from build123d import *

# Parameters (mm, degrees)
MODEL_W                      = 31.7
MODEL_H                      = 20.375
SALIENTE_EXTRUIR1_DEPTH      = 4
SALIENTE_EXTRUIR2_DEPTH      = 4
SALIENTE_EXTRUIR2_DEPTH_BACK = 4
CROQUIS3_W                   = 37.7
CROQUIS3_H                   = 26.375
CROQUIS3_W_2                 = 31.7
CROQUIS3_H_2                 = 20.375
REDONDEO1_R                  = 5
REDONDEO3_R                  = 5
CROQUIS8_W                   = 31.7
CROQUIS8_H                   = 3.000145556
CORTAR_EXTRUIR2_DEPTH        = 4
CORTAR_EXTRUIR3_DEPTH        = 4
CHAFL_N3_SIZE                = 1.5
CHAFL_N4_SIZE                = 1


with BuildPart() as part:
    # Model → Saliente-Extruir1 (new body)
    with BuildSketch(Plane.XY):
        with Locations((126.95, -64.0625)):
            Rectangle(MODEL_W, MODEL_H)
        Polygon((126.809569, -61.253776), (127.077015, -61.28391), (127.339405, -61.343798), (127.59344, -61.432689), (127.835925, -61.549464), (128.063811, -61.692654), (128.274232, -61.860459), (128.464541, -62.050768), (128.632346, -62.261189), (128.775536, -62.489075), (128.892311, -62.73156), (128.981202, -62.985595), (129.04109, -63.247985), (129.071224, -63.515431), (129.071224, -63.784569), (129.04109, -64.052015), (128.981202, -64.314405), (128.892311, -64.56844), (128.775536, -64.810925), (128.632346, -65.038811), (128.464541, -65.249232), (128.274232, -65.439541), (128.063811, -65.607346), (127.835925, -65.750536), (127.59344, -65.867311), (127.339405, -65.956202), (127.077015, -66.01609), (126.809569, -66.046224), (126.540431, -66.046224), (126.272985, -66.01609), (126.010595, -65.956202), (125.75656, -65.867311), (125.514075, -65.750536), (125.286189, -65.607346), (125.075768, -65.439541), (124.885459, -65.249232), (124.717654, -65.038811), (124.574464, -64.810925), (124.457689, -64.56844), (124.368798, -64.314405), (124.30891, -64.052015), (124.278776, -63.784569), (124.278776, -63.515431), (124.279861, -63.505804), (124.30891, -63.247985), (124.368798, -62.985595), (124.457689, -62.73156), (124.574464, -62.489075), (124.717654, -62.261189), (124.885459, -62.050768), (125.075768, -61.860459), (125.286189, -61.692654), (125.514075, -61.549464), (125.75656, -61.432689), (126.010595, -61.343798), (126.272985, -61.28391), (126.540431, -61.253776), align=None, mode=Mode.SUBTRACT)
    extrude(amount=SALIENTE_EXTRUIR1_DEPTH)

    # Croquis3 → Saliente-Extruir2 (add, two sides: drawn at the far end of the back side and taken through both)
    with BuildSketch(Plane.XY.offset(4).offset(-SALIENTE_EXTRUIR2_DEPTH_BACK)):
        with Locations((126.95, -64.0625)):
            Rectangle(CROQUIS3_W, CROQUIS3_H)
        with Locations((126.95, -64.0625)):
            Rectangle(CROQUIS3_W_2, CROQUIS3_H_2, mode=Mode.SUBTRACT)
    extrude(amount=SALIENTE_EXTRUIR2_DEPTH + SALIENTE_EXTRUIR2_DEPTH_BACK)

    # Redondeo1
    redondeo1_edges = [part.edges().sort_by_distance(p)[0] for p in [
        (108.1, -77.25, 4),
        (145.8, -77.25, 4),
    ]]
    fillet(redondeo1_edges, radius=REDONDEO1_R)

    # Redondeo3
    redondeo3_edges = [part.edges().sort_by_distance(p)[0] for p in [
        (145.8, -50.875, 4),
        (108.1, -50.875, 4),
    ]]
    fillet(redondeo3_edges, radius=REDONDEO3_R)

    # Croquis8 → Cortar-Extruir2 (cut)
    with BuildSketch(Plane.XZ.offset(53.875)):
        with Locations((126.95, 6.499927222)):
            Rectangle(CROQUIS8_W, CROQUIS8_H)
    extrude(amount=-CORTAR_EXTRUIR2_DEPTH, mode=Mode.SUBTRACT)

    # Croquis9 → Cortar-Extruir3 (cut)
    with BuildSketch(Plane.XY.offset(4)):
        with BuildLine():
            Line((115.1, -56.375), (118.625993534, -56.375))
            Line((118.625993534, -56.375), (122.824085816, -56.375))
            ThreePointArc((122.824085816, -56.375), (123.884745987, -56.814339828), (124.324085816, -57.875))
            Line((124.324085816, -57.875), (124.324085816, -58.116279303))
            ThreePointArc((124.324085816, -58.116279303), (123.884745987, -59.176939475), (122.824085816, -59.616279303))
            Line((122.824085816, -59.616279303), (118.862646904, -59.616279303))
            ThreePointArc((118.862646904, -59.616279303), (117.801986732, -60.055619131), (117.362646904, -61.116279303))
            Line((117.362646904, -61.116279303), (117.362646904, -70.15))
            ThreePointArc((117.362646904, -70.15), (116.923307076, -71.210660172), (115.862646904, -71.65))
            Line((115.862646904, -71.65), (115.1, -71.65))
            ThreePointArc((115.1, -71.65), (114.039339828, -71.210660172), (113.6, -70.15))
            Line((113.6, -70.15), (113.6, -57.875))
            ThreePointArc((113.6, -57.875), (114.039339828, -56.814339828), (115.1, -56.375))
        make_face()
        with BuildLine():
            Line((138.8, -71.65), (138.037353096, -71.65))
            ThreePointArc((138.037353096, -71.65), (136.976692924, -71.210660172), (136.537353096, -70.15))
            Line((136.537353096, -70.15), (136.537353096, -63.375))
            ThreePointArc((136.537353096, -63.375), (136.976692924, -62.314339828), (138.037353096, -61.875))
            Line((138.037353096, -61.875), (138.8, -61.875))
            ThreePointArc((138.8, -61.875), (139.860660172, -62.314339828), (140.3, -63.375))
            Line((140.3, -63.375), (140.3, -70.15))
            ThreePointArc((140.3, -70.15), (139.860660172, -71.210660172), (138.8, -71.65))
        make_face()
        with BuildLine():
            Line((130.618924081, -56.194062707), (135.761102268, -56.194062707))
            ThreePointArc((135.761102268, -56.194062707), (136.82176244, -56.633402535), (137.261102268, -57.694062707))
            Line((137.261102268, -57.694062707), (137.261102268, -57.771184154))
            ThreePointArc((137.261102268, -57.771184154), (136.82176244, -58.831844326), (135.761102268, -59.271184154))
            Line((135.761102268, -59.271184154), (130.618924081, -59.271184154))
            ThreePointArc((130.618924081, -59.271184154), (129.55826391, -58.831844326), (129.118924081, -57.771184154))
            Line((129.118924081, -57.771184154), (129.118924081, -57.694062707))
            ThreePointArc((129.118924081, -57.694062707), (129.55826391, -56.633402535), (130.618924081, -56.194062707))
        make_face()
    extrude(amount=-CORTAR_EXTRUIR3_DEPTH, mode=Mode.SUBTRACT)

    # Chaflán3
    chafl_n3_edges = [part.edges().sort_by_distance(p)[0] for p in [
        (123.884745987, -56.814339828, 4),
        (118.962042908, -56.375, 4),
        (114.039339828, -56.814339828, 4),
        (113.6, -64.0125, 4),
        (114.039339828, -71.210660172, 4),
        (115.481323452, -71.65, 4),
        (116.923307076, -71.210660172, 4),
        (117.362646904, -65.633139651, 4),
        (117.801986732, -60.055619131, 4),
        (120.84336636, -59.616279303, 4),
        (123.884745987, -59.176939475, 4),
        (124.324085816, -57.995639651, 4),
    ]]
    chamfer(chafl_n3_edges, length=CHAFL_N3_SIZE - 0.0001)  # a hair under: the kernel refuses the full size

    # Chaflán4
    chafl_n4_edges = [part.edges().sort_by_distance(p)[0] for p in [
        (139.860660172, -71.210660172, 4),
        (140.3, -66.7625, 4),
        (139.860660172, -62.314339828, 4),
        (138.418676548, -61.875, 4),
        (136.976692924, -62.314339828, 4),
        (136.537353096, -66.7625, 4),
        (136.976692924, -71.210660172, 4),
        (138.418676548, -71.65, 4),
        (136.82176244, -58.831844326, 4),
        (137.261102268, -57.73262343, 4),
        (136.82176244, -56.633402535, 4),
        (133.190013175, -56.194062707, 4),
        (129.55826391, -56.633402535, 4),
        (129.118924081, -57.73262343, 4),
        (129.55826391, -58.831844326, 4),
        (133.190013175, -59.271184154, 4),
    ]]
    chamfer(chafl_n4_edges, length=CHAFL_N4_SIZE)


solid = part.part
Source: CAD feature listing. Evaluate the final solid. Frame: model axes, mm. A direction names the side the tool comes from. Round coordinates to 2 decimals unless told otherwise and drop trailing zeros. Loops run counter-clockwise (first coordinate to the right, second up) from the corner with the lowest first, then second, coordinate; pieces in that order, holes last. Notation, with made-up numbers: M 24,78.5 L 48,78.5 A22 ccw 48,107.5 Z; hole C 10.25,87 d1. An arc over 180 degrees is marked long. Answer as CSV lines item,"result".
Q1. Reachability of faces 1 (the face through (109.526, -52.379, 4.056)), 2 (the face through (133, -56.194, 2)), 3 (the face through (120.871, -60.377, 3.261)) from +Z, -Z, +X, -X, +Y, -Y: full face, straight path, thin tool, end or side. Return the list, or none.
Verdict:
face 1,"+Z, -Z, -X, +Y"
face 2,"+Z, -Z"
face 3,"+Z"
Q2. Cut plane D-D (x = 134). Return the cut outline in (y, z) (3 decimals).
Verdict:
outline,"M -77.25,0 L -59.271,0 L -59.271,3 L -60.271,4 L -74.25,4 L -74.25,8 L -77.25,8 Z; M -56.194,0 L -50.875,0 L -50.875,5 L -53.875,5 L -53.875,4 L -55.194,4 L -56.194,3 Z"
Q3. Cut plane B-B (y = -68.25). Return the cut outline in (x, z).
Verdict:
outline,"M 108.1,0 L 113.6,0 L 113.6,2.5 L 112.1,4 L 111.1,4 L 111.1,8 L 108.1,8 Z; M 117.36,0 L 136.54,0 L 136.54,3 L 135.54,4 L 118.86,4 L 117.36,2.5 Z; M 140.3,0 L 145.8,0 L 145.8,8 L 142.8,8 L 142.8,4 L 141.3,4 L 140.3,3 Z"
Q4. Contact query for flat-ended pins moving along their axis: pin 1 (1.5 mm diameter, centred on x = 129, y = -72.5, fed in from +Z); pin 2 (12 mm diameter, centred on x = 131.5, y = -57, fed in from +Z); pin 3 (2 mm diameter, centred on y = -53.5, z = 2.5, fed in from -X); pin 4 (2 mm diameter, centred on x = 126, y = -63, fed in from -Z). Output: stop coordinate, or through.
Verdict:
pin 1,"stops at z = 4"
pin 2,"stops at z = 5"
pin 3,"stops at x = 108.29"
pin 4,"passes through"
Q5. Pull-direction query (X, two-part tool) for faces 4 (the face through (127, -67, 0)), 5 (the face through (129.547, -56.645, 1.521)), 6 (the face through (109.53, -75.75, 4.06)); classes: +X half, -X half, draft (parallel to the pull), parting line (faces both ways), or undercut.
Verdict:
face 4,"draft"
face 5,"undercut"
face 6,"-X half"
Q6. Cut plane C-C (z = 1.25). Count the separate pieces of the cut face and the enclosed holes in it, plus the area to 3 significant figures.
Verdict:
separate pieces,"1"
enclosed holes,"4"
area,"819 mm^2"
Q7. Line query: line 1 along Y through (x, z) = (121.5, 4.5) (3 decimals); line 2 along X through (y, z) = (-71.75, 4.25); line 3 along Y through (x, z) = (133, 3) (3 decimals). Output: solid intervals per line, ascending.
Verdict:
line 1,"y = -77.25 to -74.25, -53.875 to -50.875"
line 2,"x = 108.1 to 111.1, 142.8 to 145.8"
line 3,"y = -77.25 to -59.271, -56.194 to -50.875"
Q8. Cut plane A-A (x = 122). Return the cut outline in (y, z) (3 decimals), plus the area to 3 significant figures.
Verdict:
outline,"M -77.25,0 L -59.616,0 L -59.616,2.5 L -61.116,4 L -74.25,4 L -74.25,8 L -77.25,8 Z; M -56.375,0 L -50.875,0 L -50.875,5 L -53.875,5 L -53.875,4 L -54.875,4 L -56.375,2.5 Z"
area,"105 mm^2"
